The listing builds one solid part. Answer for the finished solid, in the listing's coordinates (mm). Coordinates: 2 decimals unless noted, no trailing zeros. Order: outer loops, then holes, each group sorted by start corner. A loop starts at its lowest first (then second) coordinate and runs counter-clockwise, first axis right, second up. Notation, with made-up numbers: (21.5, 26) -> (36.5, 26) arc R16 cw to (36.5, 51) -> close; hole circle Ø1 at (64, 34.5). An arc over 180 degrees is marked (long way). Return JSON: item names as keys, results as strings.
from build123d import *

# Parameters (mm, degrees)
BOSS_EXTRUDE1_DEPTH = 10
FILLET1_R           = 5
FILLET2_R           = 5
FILLET3_R           = 5
FILLET4_R           = 5


with BuildPart() as part:
    # Sketch1 → Boss-Extrude1 (new body)
    with BuildSketch(Plane.XY):
        with BuildLine():
            Line((0, 10), (0, 5))
            Line((0, 5), (3, 5))
            ThreePointArc((3, 5), (4.5, 6.5), (6, 5))
            Line((6, 5), (134, 5))
            ThreePointArc((134, 5), (135.5, 6.5), (137, 5))
            Line((137, 5), (140, 5))
            Line((140, 5), (140, 10))
            Line((140, 10), (0, 10))
        make_face()
        with BuildLine():
            Line((3, 5), (0, 5))
            Line((0, 5), (0, 0))
            Line((0, 0), (140, 0))
            Line((140, 0), (140, 5))
            Line((140, 5), (137, 5))
            ThreePointArc((137, 5), (135.5, 3.5), (134, 5))
            Line((134, 5), (6, 5))
            ThreePointArc((6, 5), (4.5, 3.5), (3, 5))
        make_face()
    extrude(amount=BOSS_EXTRUDE1_DEPTH)

    # Fillet1
    fillet1_edges = [part.edges().sort_by_distance(p)[0] for p in [
        (0, 10, 5),
    ]]
    fillet(fillet1_edges, radius=FILLET1_R)

    # Fillet2
    fillet2_edges = [part.edges().sort_by_distance(p)[0] for p in [
        (0, 0, 5),
    ]]
    fillet(fillet2_edges, radius=FILLET2_R - 0.0001)  # a hair under: the kernel refuses the full size

    # Fillet3
    fillet3_edges = [part.edges().sort_by_distance(p)[0] for p in [
        (140, 10, 5),
    ]]
    fillet(fillet3_edges, radius=FILLET3_R)

    # Fillet4
    fillet4_edges = [part.edges().sort_by_distance(p)[0] for p in [
        (140, 0, 5),
    ]]
    fillet(fillet4_edges, radius=FILLET4_R - 0.0001)  # a hair under: the kernel refuses the full size


solid = part.part
1. This flat-tipped pin is pushed along its axis until it touches: pin 1 Ø3 at (y, z) = (2.5, 5) entering from -X. Where does it stop, or does it pass through?
Answer block:
{"pin 1": "stops at x = 0.1"}
2. The part is cut by section A-A on z = 4. Give the number of separate pieces and of enclosed holes in the cut face, and give its area (3 significant figures).
Answer block:
{"separate pieces": "1", "enclosed holes": "2", "area": "1,360 mm2"}
3. Determine the mould class of faces 1 (the face through (6, 5, 5)), 2 (the face through (69, 5, 0)), 3 (the face through (71, 10, 5)) for opening direction Y: pulls with the +Y half, pulls with the -Y half, needs draft (parallel to the pull), parting line crosses it, or undercut.
Answer block:
{"face 1": "undercut", "face 2": "needs draft", "face 3": "pulls with the +Y half"}
4. The part is cut by section B-B on y = 1.5. Give the vertices of the cut face in (x, z), and give its area (3 significant figures).
Answer block:
{"outline": "(1.43, 0) -> (138.57, 0) -> (138.57, 10) -> (1.43, 10) -> close", "area": "1,370 mm2"}
5. Consider line 1 (X direction, y = 5.25, z = 5); line 2 (Y direction, x = 4.5, z = 7); line 3 (X direction, y = 4.25, z = 3). Determine where each line is inside the solid, lowest interval first. Write a range as from..to.
Answer block:
{"line 1": "x = 0.01..3.02, 5.98..134.02, 136.98..139.99", "line 2": "y = 0.03..3.5, 6.5..9.97", "line 3": "x = 0.06..3.2, 5.8..134.2, 136.8..139.94"}
